Check sheet for the modelled part. Datum: model origin and axes. Units: mm. Coordinates: 2 decimals unless noted, no trailing zeros. Write each loop counter-clockwise with the first axis right and the second up, starting at its lowest first coordinate (ties: lowest second). Pieces come first, ordered by that corner, then holes. Notation, with made-up numbers: (65.25, -38) - (105.25, -38) arc R10 cw to (105.25, -19) - close; hole circle Ø1 at (22, 86). An arc over 180 degrees is marked (long way). Use one line per item in the form item = value. Start each with the question number.
1. Go/stop test with flat-tipped pins: pin 1 Ø3 at (x, y) = (54, 6) entering from +Z; pin 2 Ø12 at (x, y) = (47, -16.5) entering from +Z. Record where each tip stops, or that it passes through.
2. Cross-section at A-A on y = 19. Record the boundary of the cut face in (x, z), then the cut area to 3 significant figures.
3. Scan lines: line 1 along X through (y, z) = (17, -15.5); line 2 along Z through (x, y) = (32, 10); line 3 along Z through (x, y) = (52, 8). Record each from-to range of solid material in increasing order.
4. Cross-section at B-B on x = 14. Record the boundary of the cut face in (y, z).
Autodesk Inventor part; units mm, degrees
ref_plane "工作平面1" through (10, 22, 0) normal (-0.3499, -0.6624, -0.6624) x (0.8842, 0, -0.4671)
ref_plane "YZ Plane" through (0, 0, 0) normal (1, 0, 0) x (0, 1, 0)
ref_plane "XZ Plane" through (0, 0, 0) normal (0, 1, 0) x (-1, 0, 0)
sketch "草圖1" plane through (0, 0, 0) normal (0, 1, 0) x (-1, 0, 0)
  line L0 (0, 0) -> (-63, 0)
  line L1 (-63, 0) -> (-63, -38)
  line L2 (-63, -38) -> (0, -38)
  line L3 (0, -38) -> (0, 0)
  dimension "d0" = 63
  dimension "d1" = 38
extrude "擠出1" add sketch "草圖1" along normal mid plane 44
sketch "草圖2" plane through (0, 22, 0) normal (0, 1, 0) x (1, 0, 0)
  line L0 (0, 0) -> (63, 0)
  line L1 (10, 0) -> (63, 8)
  line L2 (63, 0) -> (63, 38)
  dimension "d4" = 10
  dimension "d5" = 30
extrude "擠出2" cut sketch "草圖2" against normal blind 60
sketch "草圖3" plane through (63, -22, -38) normal (1, 0, 0) x (0, 0, -1)
  line L0 (-30, 24) -> (-10, 44)
  line L1 (0, 44) -> (-38, 44)
  line L2 (-30, 44) -> (-30, 0)
  point P0 (-38, 22)
  point P1 (-30, 2)
  dimension "d8" = 20
  dimension "d9" = 20
ref_plane "工作平面1" through (10, 22, 0) normal (-0.3499, -0.6624, -0.6624) x (0.8842, 0, -0.4671)
sketch "草圖4" plane through (10, 22, 0) normal (-0.3499, -0.6624, -0.6624) x (0.8842, 0, -0.4671)
  line L0 (-15.1543, -12.3218) -> (93.717, -12.3218)
  line L1 (93.717, -12.3218) -> (93.717, 28.8166)
  line L2 (93.717, 28.8166) -> (-15.1543, 28.8166)
  line L3 (-15.1543, 28.8166) -> (-15.1543, -12.3218)
  point P0 (-8.8419, 13.3872)
extrude "擠出3" cut sketch "草圖4" against normal blind 40
mirror "鏡射1" about plane through (0, 0, 0) normal (0, 1, 0) of "擠出3"
properties part number "54"
Final values:
q1.pin_1 = -6.42
q1.pin_2 = -7.26
q2.outline = (0, -38) - (63, -38) - (63, -25) - (17.94, -1.2) - (10, 0) - (0, 0) - close
q2.area = 1,800 mm²
q3.line_1 = 0 to 48.8
q3.line_2 = -38 to -3.32
q3.line_3 = -38 to -8.19
q4.outline = (-22, -38) - (22, -38) - (22, -2.12) - (20.49, -0.6) - (-20.49, -0.6) - (-22, -2.12) - close
